Build history of the part. All positions in model axes, mm. Coordinates: 2 decimals unless noted, no trailing zeros. Write each loop counter-clockwise with the first axis right and the second up, starting at its lowest first coordinate (ties: lowest second). Pieces come first, ordered by that corner, then holes. Notation, with made-up numbers: (69, 43.5) -> (106, 43.5) arc R35 cw to (106, 82.5) -> close; hole circle Ø1 at (7, -31). An arc over 180 degrees is marked (long way). Write each question's results on one line, items separated by ' | '. Start each with the question number.
Q1. Drop flat-ended pins along their axis: pin 1 Ø0.8 at (x, z) = (26, 1) entering from +Y; pin 2 Ø0.6 at (y, z) = (15, 1) entering from -X; pin 3 Ø2 at (x, y) = (61.5, 21.5) entering from +Z; pin 4 Ø1.1 at (y, z) = (53, 1) entering from -X. Give the stop position or say it passes through.
Q2. Drill centre lines: line 1 (X direction, y = 42.5, z = 0.6); line 2 (X direction, y = 34.5, z = 1.2); line 3 (Y direction, x = 52, z = 1.65). Where is each one in solid material? Low to high.
Q3. Saw through at B-B on y = 39.5. Give the cut face in (x, z).
Q4. Saw through at A-A on x = 48. Give the cut face in (y, z), and give its area (3 significant figures).
Q5. Saw through at C-C on x = 31. Give the cut face in (y, z).
Q6. Saw through at D-D on y = 50. Give the cut face in (x, z).
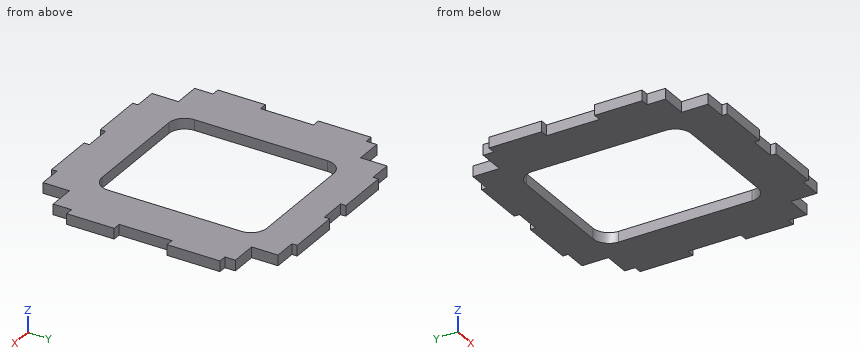
from build123d import *

# Parameters (mm, degrees)
EXTRUDE_1_DEPTH = 2


with BuildPart() as part:
    # Model → 凸台-拉伸1 (new body)
    with BuildSketch(Plane.XY):
        Polygon((31.698795353, 52.657311482), (35.978795353, 52.657311482), (35.978795353, 53.657667188), (45.978795353, 53.657667188), (45.978795353, 52.657311482), (50.978795353, 52.657311482), (50.978795353, 53.657667188), (60.978795353, 53.657667188), (60.978795353, 52.657311482), (65.258795353, 52.657311482), (65.258795353, 47.657311482), (70.258795353, 47.657311482), (70.258795353, 45.667311482), (71.758795353, 45.667311482), (71.758795353, 35.667311482), (70.258795353, 35.667311482), (70.258795353, 25.667311482), (71.758795353, 25.667311482), (71.758795353, 16.667311482), (70.258795353, 16.667311482), (70.258795353, 15.517311482), (70.258795353, 13.201678386), (65.258795353, 13.201678386), (65.258795353, 8.201678386), (60.978795353, 8.201678386), (60.978795353, 7.20132268), (50.978795353, 7.20132268), (50.978795353, 8.201678386), (45.978795353, 8.201678386), (45.978795353, 7.20132268), (35.978795353, 7.20132268), (35.978795353, 8.201678386), (31.698795353, 8.201678386), (31.698795353, 13.201678386), (26.698795353, 13.201678386), (26.698795353, 15.517311482), (26.698795353, 16.667311482), (25.198795353, 16.667311482), (25.198795353, 25.667311482), (26.698795353, 25.667311482), (26.698795353, 35.667311482), (25.198795353, 35.667311482), (25.198795353, 45.667311482), (26.698795353, 45.667311482), (26.698795353, 47.657311482), (31.698795353, 47.657311482), align=None)
        with BuildLine():
            Line((58.847883072, 46.60843734), (38.287883072, 46.60843734))
            ThreePointArc((38.287883072, 46.60843734), (36.166562728, 45.729757683), (35.287883072, 43.60843734))
            Line((35.287883072, 43.60843734), (35.287883072, 18.43843734))
            ThreePointArc((35.287883072, 18.43843734), (36.166562728, 16.317116996), (38.287883072, 15.43843734))
            Line((38.287883072, 15.43843734), (58.847883072, 15.43843734))
            ThreePointArc((58.847883072, 15.43843734), (60.969203415, 16.317116996), (61.847883072, 18.43843734))
            Line((61.847883072, 18.43843734), (61.847883072, 43.60843734))
            ThreePointArc((61.847883072, 43.60843734), (60.969203415, 45.729757683), (58.847883072, 46.60843734))
        make_face(mode=Mode.SUBTRACT)
    extrude(amount=EXTRUDE_1_DEPTH)


solid = part.part
Returned:
1) pin 1: stops at y = 45.67 | pin 2: stops at x = 26.7 | pin 3: stops at z = 2 | pin 4: stops at x = 31.7
2) line 1: x = 25.2 to 35.29, 61.85 to 71.76 | line 2: x = 26.7 to 35.29, 61.85 to 70.26 | line 3: y = 7.2 to 15.44, 46.61 to 53.66
3) outline: (25.2, 0) -> (35.29, 0) -> (35.29, 2) -> (25.2, 2) -> close; (61.85, 0) -> (71.76, 0) -> (71.76, 2) -> (61.85, 2) -> close
4) outline: (8.2, 0) -> (15.44, 0) -> (15.44, 2) -> (8.2, 2) -> close; (46.61, 0) -> (52.66, 0) -> (52.66, 2) -> (46.61, 2) -> close | area: 26.6 mm2
5) outline: (13.2, 0) -> (47.66, 0) -> (47.66, 2) -> (13.2, 2) -> close
6) outline: (31.7, 0) -> (65.26, 0) -> (65.26, 2) -> (31.7, 2) -> close
